Model file for the job. Use its own axes, mm. Round coordinates to 2 decimals unless told otherwise and drop trailing zeros. Loops run counter-clockwise (first coordinate to the right, second up) from the corner with the lowest first, then second, coordinate; pieces in that order, holes last. Notation, with made-up numbers: M 70,-38 L 119,-38 A28 ccw 119,1 Z; hole C -32.5,-21 d3. An arc over 180 degrees is marked long. Use a Markdown table: item, result. Add a question column.
Item 1: Saw through at B-B on z = 1.4. Give the number of separate pieces and of enclosed holes in the cut face, then the cut area to 3 significant figures.
Item 2: Pin check, flat tips, straight feed: P1, Ø5, axis at x = 32.5, y = 0, coming from the -Z side; P2, Ø3.5, axis at x = 100, y = 29, coming from the +Z side. Stop position of each tip, or through.
Item 3: Saw through at D-D on x = 98.5. Write the cut outline in (y, z).
Item 4: Saw through at A-A on x = -32.5. Write the cut outline in (y, z).
Item 5: Wall check: L1, parallel to Y at x = -97.5, z = 1.6; L2, parallel to X at y = 30, z = 0.3; L3, parallel to Y at x = 32.5, z = -0.3. Give the ranges that are in metal, low to high. Write a range as from..to.
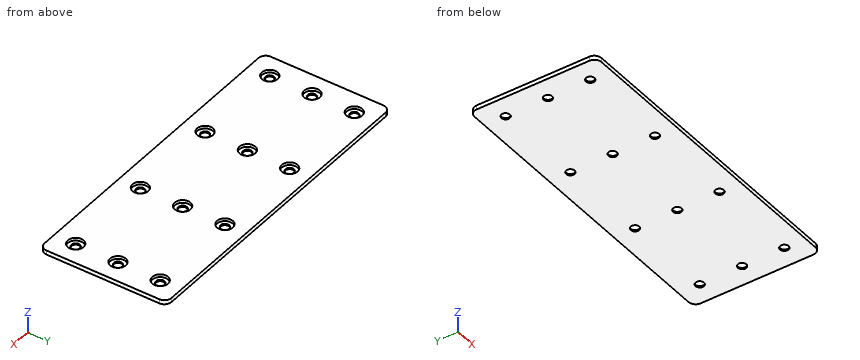
```python
from build123d import *

# Parameters (mm, degrees)
SKETCH001_W     = 225
SKETCH001_H     = 90
PAD_DEPTH       = 2
PAD_DEPTH_BACK  = 1
SKETCH_R        = 5.6
POCKET_DEPTH    = 2.001
SKETCH004_R     = 3
POCKET001_DEPTH = 1.001
FILLET_R        = 5


with BuildPart() as part:
    # Sketch001 → Pad (new body, two sides)
    with BuildSketch(Plane.XY) as pad_sk:
        Rectangle(SKETCH001_W, SKETCH001_H)
    extrude(amount=PAD_DEPTH)
    extrude(pad_sk.sketch, amount=-PAD_DEPTH_BACK)

    # Sketch → Pocket (cut, through all)
    with BuildSketch(Plane.XY):
        with Locations((-97.5, 30)):
            Circle(SKETCH_R)
        with Locations((-32.5, 30)):
            Circle(SKETCH_R)
        with Locations((32.5, 30)):
            Circle(SKETCH_R)
        with Locations((97.5, 30)):
            Circle(SKETCH_R)
        with Locations((-97.5, 0)):
            Circle(SKETCH_R)
        with Locations((-32.5, 0)):
            Circle(SKETCH_R)
        with Locations((32.5, 0)):
            Circle(SKETCH_R)
        with Locations((97.5, 0)):
            Circle(SKETCH_R)
        with Locations((-97.5, -30)):
            Circle(SKETCH_R)
        with Locations((-32.5, -30)):
            Circle(SKETCH_R)
        with Locations((32.5, -30)):
            Circle(SKETCH_R)
        with Locations((97.5, -30)):
            Circle(SKETCH_R)
    extrude(amount=POCKET_DEPTH, mode=Mode.SUBTRACT)

    # Sketch004 → Pocket001 (cut, through all)
    with BuildSketch(Plane.XY):
        with Locations((-97.5, 30)):
            Circle(SKETCH004_R)
        with Locations((-32.5, 30)):
            Circle(SKETCH004_R)
        with Locations((32.5, 30)):
            Circle(SKETCH004_R)
        with Locations((97.5, 30)):
            Circle(SKETCH004_R)
        with Locations((-97.5, 0)):
            Circle(SKETCH004_R)
        with Locations((-32.5, 0)):
            Circle(SKETCH004_R)
        with Locations((32.5, 0)):
            Circle(SKETCH004_R)
        with Locations((97.5, 0)):
            Circle(SKETCH004_R)
        with Locations((-97.5, -30)):
            Circle(SKETCH004_R)
        with Locations((-32.5, -30)):
            Circle(SKETCH004_R)
        with Locations((32.5, -30)):
            Circle(SKETCH004_R)
        with Locations((97.5, -30)):
            Circle(SKETCH004_R)
    extrude(amount=-POCKET001_DEPTH, mode=Mode.SUBTRACT)

    # Fillet
    fillet_edges = [part.edges().sort_by_distance(p)[0] for p in [
        (-112.5, -45, 0.5),
        (-112.5, 45, 0.5),
        (112.5, -45, 0.5),
        (112.5, 45, 0.5),
    ]]
    fillet(fillet_edges, radius=FILLET_R)


solid = part.part
```
Entries:
| question | item | result |
|---|---|---|
| 1 | separate pieces | 1 |
| 1 | enclosed holes | 12 |
| 1 | area | 19,000 mm2 |
| 2 | P1 | through |
| 2 | P2 | z = 0 |
| 3 | outline | M -45,-1 L -32.83,-1 L -32.83,0 L -35.51,0 L -35.51,2 L -45,2 Z; M -27.17,-1 L -2.83,-1 L -2.83,0 L -5.51,0 L -5.51,2 L -24.49,2 L -24.49,0 L -27.17,0 Z; M 2.83,-1 L 27.17,-1 L 27.17,0 L 24.49,0 L 24.49,2 L 5.51,2 L 5.51,0 L 2.83,0 Z; M 32.83,-1 L 45,-1 L 45,2 L 35.51,2 L 35.51,0 L 32.83,0 Z |
| 4 | outline | M -45,-1 L -33,-1 L -33,0 L -35.6,0 L -35.6,2 L -45,2 Z; M -27,-1 L -3,-1 L -3,0 L -5.6,0 L -5.6,2 L -24.4,2 L -24.4,0 L -27,0 Z; M 3,-1 L 27,-1 L 27,0 L 24.4,0 L 24.4,2 L 5.6,2 L 5.6,0 L 3,0 Z; M 33,-1 L 45,-1 L 45,2 L 35.6,2 L 35.6,0 L 33,0 Z |
| 5 | L1 | -45..-35.6, -24.4..-5.6, 5.6..24.4, 35.6..45 |
| 5 | L2 | -112.5..-103.1, -91.9..-38.1, -26.9..26.9, 38.1..91.9, 103.1..112.5 |
| 5 | L3 | -45..-33, -27..-3, 3..27, 33..45 |
